Can you work these out from the model? Positions are in its coordinate system, mm. A direction names the side the tool comes from. Give positions to 0.01 mm unless a question says otherwise; leave off trailing zeros. Order: outer loops, then holes, each group sorted by start corner. A loop starts at its lowest first (then second) coordinate and runs counter-clockwise, first axis right, second up. Notation, with made-up numbers: M 50.5,52.5 L 83.5,52.5 A22 cw 83.5,72.5 Z; hole C 78,26.25 d4. An arc over 180 degrees is marked long. One line per question, with ' | ' between items. Start each with the question number.
1) Thinking about a two-plate mould opening in Y: for faces 3 (the flat face through (13.1, -4.2, 15)), 4 (the cylindrical face through (4.336, 19.524, 7.605)), 5 (the cylindrical face through (1.99, -8.97, 5.92)), which applies, +Y half, -Y half, draft (parallel to the pull), parting line (faces both ways), or undercut?
2) If we section it at D-D, the plane x = 17: Please give me the cut outline in (y, z), plus the area to 3 significant figures.
3) Please list where these lines run through material, in increasing order: line 1 along Y through (x, z) = (0, 8); line 2 along Z through (x, y) = (14, 5); line 3 along Z through (x, y) = (1, -14.5). Write a range as [from, to].
4) For faces 1 (the cylindrical face through (2.01, -9.15, 28.86)), 2 (the flat face through (0, 0, 12)), which set-ups out of +Z, -Z, +X, -X, +Y, -Y let a thin tool reach every point of the face, with its end or its side?
5) If we section it at C-C, the plane x = -16: Please give me the cut outline in (y, z).
6) If we section it at A-A, the plane x = 10: Please give me the cut outline in (y, z), plus the area to 3 significant figures.
7) I'm going to push flat-ended pins straight in: pin 1 Ø3 at (y, z) = (-20.5, 16.5) entering from -X; pin 2 Ø14.5 at (x, y) = (2.5, 1) entering from -Z; pin 3 Ø14.5 at (x, y) = (0, 0) entering from -Z; pin 4 Ø8 at (y, z) = (-6.5, 23) entering from +X. Where does each tip first touch, or does it pass through?
8) If we section it at B-B, the plane z = 16: Please give me the cut outline in (x, y).
Autodesk Inventor part; units mm, degrees
ref_plane "YZ Plane" through (0, 0, 0) normal (1, 0, 0) x (0, 1, 0)
ref_plane "XZ Plane" through (0, 0, 0) normal (0, 1, 0) x (-1, 0, 0)
ref_plane "XY Plane" through (0, 0, 0) normal (0, 0, 1) x (1, 0, 0)
sketch "Sketch1" plane through (0, 0, 0) normal (0, 1, 0) x (-1, 0, 0)
  line L0 (0, 0) -> (20, 0)
  line L1 (20, 0) -> (20, 15)
  line L2 (20, 15) -> (13.5, 15)
  line L3 (0, 25) -> (0, 0)
  line L4 (0, 0) -> (0, 15.843) construction
  line L5 (0, 25) -> (13.5, 25) construction
  line L6 (13.5, 25) -> (13.5, 15) construction
  line L7 (0, 0) -> (0, -31.0844) construction
  arc A0 (13.5, 15) -> (0, 25) centre (0, 10.8875) ccw
  dimension "d0" = 20
  dimension "d1" = 15
  dimension "d3" = 25
  dimension "d4" = 13.5
revolve "Revolution1" add sketch "Sketch1" angle 360 about axis through (0, 0, 0) along (0, 0, -1)
sketch "Sketch2" plane through (0, 0, 0) normal (1, 0, 0) x (0, 1, 0)
  line L0 (0, 19) -> (-45.3208, 41.1044) construction
  line L1 (0, 19) -> (-38.3392, 19) construction
  line L2 (-20, 0) -> (20, 0) construction
  line L3 (0, 19) -> (0, 0) construction
  line L4 (0, 19) -> (2.3014, 23.7187)
  line L5 (2.3014, 23.7187) -> (-14.3262, 31.8285)
  line L6 (-14.3262, 31.8285) -> (-14.8742, 30.705)
  line L7 (-14.8742, 30.705) -> (-40.9392, 43.4178)
  line L8 (-40.9392, 43.4178) -> (-42.6927, 39.8226)
  line L9 (-42.6927, 39.8226) -> (0, 19)
  dimension "d6" = 19
  dimension "d7" = 26
  dimension "d8" = 18.5
  dimension "d9" = 29
  dimension "d10" = 4
  dimension "d11" = 5.25
revolve "Revolution2" add sketch "Sketch2" angle 360 about axis through (0, 0, 19) along (0, -0.898794, 0.4383711)
sketch "Sketch3" plane through (0, 0, 0) normal (0, 0, -1) x (-1, 0, 0)
  circle A0 centre (0, 0) radius 9.1875
  dimension "d13" = 18.375
extrude "Extrusion1" cut sketch "Sketch3" against normal blind 12
properties part number "waterbottle_lid"
Results found:
1) face 3: draft | face 4: parting line | face 5: undercut
2) outline: M -10.54,0 L 10.54,0 L 10.54,15 L -10.54,15 Z | area: 316 mm²
3) line 1: y = [-20, -9.19], [9.19, 20] | line 2: z = [0, 15] | line 3: z = [0, 15], [20.34, 31.47]
4) face 1: none | face 2: -Z
5) outline: M -12,0 L 12,0 L 12,15 L -12,15 Z
6) outline: M -17.32,0 L 17.32,0 L 17.32,15 L 9.07,15 A9.96 ccw -9.07,15 L -17.32,15 Z | area: 596 mm²
7) pin 1: passes through | pin 2: stops at z = 0 | pin 3: stops at z = 12 | pin 4: stops at x = 10.21
8) outline: C 0,0 d26.31
